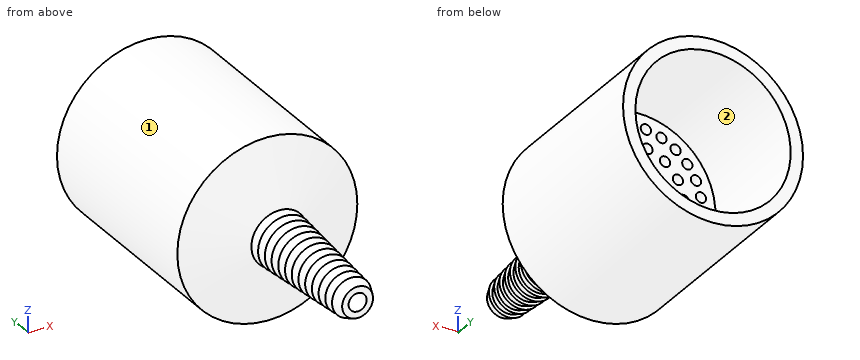
```python
from build123d import *

# Parameters (mm, degrees)
SKETCH_1_R          = 17.5
EXTRUDE_1_DEPTH     = 40
SKETCH_2_R          = 15.1
CUT_EXTRUDE_1_DEPTH = 35
SKETCH_5_R          = 1.75
CUT_EXTRUDE_2_DEPTH = 71
SKETCH_8_R          = 17.5
EXTRUDE_2_DEPTH     = 5
SKETCH_11_R         = 1
CUT_EXTRUDE_3_DEPTH = 5


with BuildPart() as part:
    # 草图1 → 凸台-拉伸1 (new body)
    with BuildSketch(Plane(origin=(0, 0, 0), x_dir=(1, 0, 0), z_dir=(0, 1, 0))):
        Circle(SKETCH_1_R)
    extrude(amount=EXTRUDE_1_DEPTH)

    # 草图2 → 切除-拉伸1 (cut)
    with BuildSketch(Plane(origin=(0, 40, 0), x_dir=(1, 0, 0), z_dir=(0, 1, 0))):
        Circle(SKETCH_2_R)
    extrude(amount=-CUT_EXTRUDE_1_DEPTH, mode=Mode.SUBTRACT)

    # 草图4 → 旋转1 (revolve)
    with BuildSketch(Plane.XY):
        Polygon((0, 0), (0, -30), (3, -30), (3.8, -28), (3.139853624, -28), (3.939512947, -26.004871899), (3.279366571, -26.004871899), (4.079025895, -24.009743799), (3.418879519, -24.009743799), (4.218538842, -22.014615698), (3.558392466, -22.014615698), (4.35805179, -20.019487598), (3.697905414, -20.019487598), (4.497564737, -18.024359497), (3.837418361, -18.024359497), (4.637077685, -16.029231397), (3.976931309, -16.029231397), (4.776590632, -14.034103296), (4.116444256, -14.034103296), (4.91610358, -12.038975196), (4.255957204, -12.038975196), (5.055616527, -10.043847095), (4.395470151, -10.043847095), (5.195129475, -8.048718995), (4.534983099, -8.048718995), (5.334642422, -6.053590894), (4.674496046, -6.053590894), (5.47415537, -4.058462794), (4.814008994, -4.058462794), (17.5, 0), align=None)
    revolve(axis=Axis((0, 0, 0), (0, -1, 0)))

    # 草图5 → 切除-拉伸2 (cut, through all)
    with BuildSketch(Plane.XZ.offset(30)):
        Circle(SKETCH_5_R)
    extrude(amount=-CUT_EXTRUDE_2_DEPTH, mode=Mode.SUBTRACT)

    # 草图8 → 凸台-拉伸2 (add)
    with BuildSketch(Plane(origin=(0, 10, 0), x_dir=(1, 0, 0), z_dir=(0, 1, 0))):
        Circle(SKETCH_8_R)
    extrude(amount=EXTRUDE_2_DEPTH)

    # 草图11 → 切除-拉伸3 (cut)
    with BuildSketch(Plane(origin=(0, 15, 0), x_dir=(1, 0, 0), z_dir=(0, 1, 0))):
        with Locations((0, 9)):
            Circle(SKETCH_11_R)
        with Locations((3.660629788, 8.221909119)):
            Circle(SKETCH_11_R)
        with Locations((6.688303429, 6.022175457)):
            Circle(SKETCH_11_R)
        with Locations((8.559508647, 2.781152949)):
            Circle(SKETCH_11_R)
        with Locations((8.950697058, -0.940756169)):
            Circle(SKETCH_11_R)
        with Locations((7.794228634, -4.5)):
            Circle(SKETCH_11_R)
        with Locations((5.290067271, -7.281152949)):
            Circle(SKETCH_11_R)
        with Locations((1.871205217, -8.803328407)):
            Circle(SKETCH_11_R)
        with Locations((-1.871205217, -8.803328407)):
            Circle(SKETCH_11_R)
        with Locations((-5.290067271, -7.281152949)):
            Circle(SKETCH_11_R)
        with Locations((-7.794228634, -4.5)):
            Circle(SKETCH_11_R)
        with Locations((-8.950697058, -0.940756169)):
            Circle(SKETCH_11_R)
        with Locations((-8.559508647, 2.781152949)):
            Circle(SKETCH_11_R)
        with Locations((-6.688303429, 6.022175457)):
            Circle(SKETCH_11_R)
        with Locations((-3.660629788, 8.221909119)):
            Circle(SKETCH_11_R)
        with Locations((0, 12.5)):
            Circle(SKETCH_11_R)
        with Locations((3.10862359, 12.107289514)):
            Circle(SKETCH_11_R)
        with Locations((6.021920926, 10.953833501)):
            Circle(SKETCH_11_R)
        with Locations((8.556838824, 9.112107843)):
            Circle(SKETCH_11_R)
        with Locations((10.554099069, 6.697834937)):
            Circle(SKETCH_11_R)
        with Locations((11.888206454, 3.86271243)):
            Circle(SKETCH_11_R)
        with Locations((12.475334105, 0.784881494)):
            Circle(SKETCH_11_R)
        with Locations((12.278590634, -2.342266432)):
            Circle(SKETCH_11_R)
        with Locations((11.310338156, -5.322241145)):
            Circle(SKETCH_11_R)
        with Locations((9.631415535, -7.967799872)):
            Circle(SKETCH_11_R)
        with Locations((7.347315654, -10.11271243)):
            Circle(SKETCH_11_R)
        with Locations((4.601556909, -11.622206074)):
            Circle(SKETCH_11_R)
        with Locations((1.56666542, -12.401433766)):
            Circle(SKETCH_11_R)
        with Locations((-1.56666542, -12.401433766)):
            Circle(SKETCH_11_R)
        with Locations((-4.601556909, -11.622206074)):
            Circle(SKETCH_11_R)
        with Locations((-7.347315654, -10.11271243)):
            Circle(SKETCH_11_R)
        with Locations((-9.631415535, -7.967799872)):
            Circle(SKETCH_11_R)
        with Locations((-11.310338156, -5.322241145)):
            Circle(SKETCH_11_R)
        with Locations((-12.278590634, -2.342266432)):
            Circle(SKETCH_11_R)
        with Locations((-12.475334105, 0.784881494)):
            Circle(SKETCH_11_R)
        with Locations((-11.888206454, 3.86271243)):
            Circle(SKETCH_11_R)
        with Locations((-10.554099069, 6.697834937)):
            Circle(SKETCH_11_R)
        with Locations((-8.556838824, 9.112107843)):
            Circle(SKETCH_11_R)
        with Locations((-6.021920926, 10.953833501)):
            Circle(SKETCH_11_R)
        with Locations((-3.10862359, 12.107289514)):
            Circle(SKETCH_11_R)
    extrude(amount=-CUT_EXTRUDE_3_DEPTH, mode=Mode.SUBTRACT)


solid = part.part
```
Source: CAD feature listing. Evaluate the final solid. Frame: model axes, mm. Face numbers are marked on the shaded views. Coordinates: 2 decimals unless noted, no trailing zeros. Loops run counter-clockwise (first coordinate to the right, second up) from the corner with the lowest first, then second, coordinate; pieces in that order, holes last. Notation, with made-up numbers: (-37.75, 58) -> (-24.75, 58) arc R18 cw to (-24.75, 73) -> close; hole circle Ø11 at (3, 79.25). An arc over 180 degrees is marked (long way). One line per item, written item: value. Start each with the question number.
Q1. Section query A-A, the plane y = -7. Return the cut outline in (x, z).
Q2. Mould query, pull axis X, two halves, no side actions, for the marked faces 1 and 2. Classes: pulls with the +X half, pulls with the -X half, needs draft (parallel to the pull), parting line crosses it, or undercut.
Q3. Line query: line 1 along Z through (x, y) = (0, 11.85); line 2 along X through (y, z) = (13, 11.5); line 3 along X through (y, z) = (11, -12). Output: solid intervals per line, ascending.
Q4. Contact query for flat-ended pins moving along their axis: P1, Ø6, axis at x = -2, z = 0.5, coming from the +Y side; P2, Ø1.2, axis at x = -11.31, z = 5.32, coming from the +Y side; P3, Ø2.5, axis at x = -1.57, z = 12.4, coming from the -Y side. Output: stop coordinate, or through.
Results:
1. outline: circle Ø9.91 at (0, 0); hole circle Ø3.5 at (0, 0)
2. face 1: parting line crosses it
2. face 2: undercut
3. line 1: -17.5 to -13.5, -11.5 to -10, -8 to 17.5
3. line 2: -13.19 to -5.59, -3.61 to -2, -1.13 to 1.13, 2 to 3.61, 5.59 to 13.19
3. line 3: -12.74 to -4.1, -2.11 to -0.87, 0.87 to 2.11, 4.1 to 12.74
4. P1: y = 15
4. P2: y = 5
4. P3: y = -2
